The drawing under review shows one solid part. Ordinate dimensions are in mm from its lowest x, y, z. A direction names the side the tool comes from. Coordinates: 2 decimals unless noted, no trailing zeros. Loops run counter-clockwise (first coordinate to the right, second up) from the corner with the lowest first, then second, coordinate; pieces in that order, holes last. Notation, with made-up numbers: M -24.75,-26 L 22.25,-26 A12 ccw 22.25,-14 Z; hole C 64,55.25 d4. An arc over 180 degrees is marked long. Return JSON: item names as keys, results as strings.
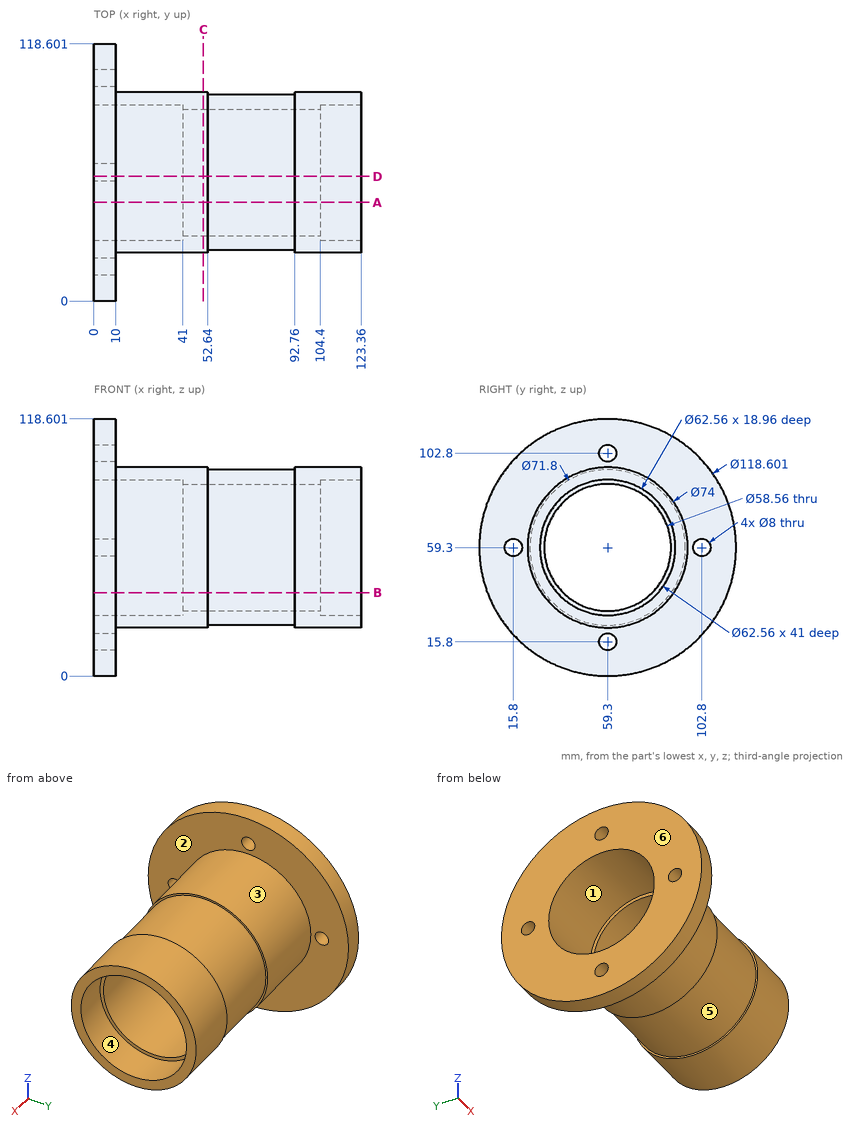
1. Add section C-C on x = 50.5. Give the boundary of the cut face in (y, z), plus the area to 3 significant figures.
Check values:
{"outline": "C 59.3,59.3 d74; hole C 59.3,59.3 d58.56", "area": "1,610 mm²"}
2. Add section D-D on y = 57.5. State how many separate pieces and enclosed holes the cut face has, plus the area to 3 significant figures.
Check values:
{"separate pieces": "4", "enclosed holes": "0", "area": "1,880 mm²"}
3. To check wall thickness, follow line 1 (Z direction, x = 87, y = 34.5) (1 decimal); line 2 (X direction, y = 29, z = 105); line 3 (Y direction, x = 114, z = 57.5) (1 decimal). State the ranges of each line that lie inside material, in increasing order.
Check values:
{"line 1": "33.3 to 43.7, 74.9 to 85.3", "line 2": "0 to 10", "line 3": "22.3 to 28.1, 90.5 to 96.3"}
4. Add section B-B on z = 38.5. Give the boundary of the cut face in (x, y), plus the area to 3 significant figures.
Check values:
{"outline": "M 0,3.77 L 10,3.77 L 10,28.7 L 52.64,28.7 L 52.64,30.04 L 92.76,30.04 L 92.76,28.7 L 123.36,28.7 L 123.36,35.94 L 104.4,35.94 L 104.4,38.69 L 41,38.69 L 41,35.94 L 0,35.94 Z; M 0,82.66 L 41,82.66 L 41,79.91 L 104.4,79.91 L 104.4,82.66 L 123.36,82.66 L 123.36,89.9 L 92.76,89.9 L 92.76,88.56 L 52.64,88.56 L 52.64,89.9 L 10,89.9 L 10,114.83 L 0,114.83 Z", "area": "2,530 mm²"}
5. Insertion check: pin 1 Ø8 at (x, y) = (13, 93) entering from +Z; pin 2 Ø22 at (y, z) = (41, 57.5) entering from +X; pin 3 Ø6 at (x, z) = (72, 55.5) entering from -Y; pin 4 Ø6.5 at (y, z) = (102.8, 59.3) entering from +X. Each pin has a flat end and moves straight along its axis. Give the tip position at first contact, or say it passes through.
Check values:
{"pin 1": "z = 109.82", "pin 2": "x = 104.4", "pin 3": "y = 23.41", "pin 4": "through"}
6. The part is to be moulded in two halves that separate along Y. For the marked faces 1, 2 and 3, say which applies: released by +Y, released by -Y, zero draft, split by the parting line, or undercut.
Check values:
{"face 1": "undercut", "face 2": "zero draft", "face 3": "split by the parting line"}
7. Add section A-A on y = 45.5. Give the boundary of the cut face in (x, z).
Check values:
{"outline": "M 0,1.63 L 10,1.63 L 10,24.97 L 52.64,24.97 L 52.64,26.16 L 92.76,26.16 L 92.76,24.97 L 123.36,24.97 L 123.36,31.23 L 104.4,31.23 L 104.4,33.48 L 41,33.48 L 41,31.23 L 0,31.23 Z; M 0,87.37 L 41,87.37 L 41,85.12 L 104.4,85.12 L 104.4,87.37 L 123.36,87.37 L 123.36,93.63 L 92.76,93.63 L 92.76,92.44 L 52.64,92.44 L 52.64,93.63 L 10,93.63 L 10,116.97 L 0,116.97 Z"}
8. Machinability: for the marked faces 4, 5 and 6, which of the approach directions +Z, -Z, +X, -X, +Y, -Y give a long, thin tool a straight path to every point of the face, cutting with its end or side? Answer none if there is none.
Check values:
{"face 4": "+X", "face 5": "none", "face 6": "+Z, -Z, -X, +Y, -Y"}
